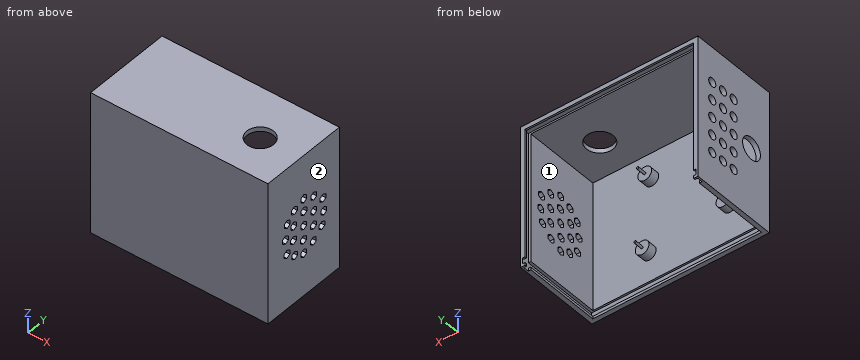
from build123d import *

# Parameters (mm, degrees)
SKETCH1_W           = 200
SKETCH1_H           = 160
BOSS_EXTRUDE1_DEPTH = 100
SHELL2_T            = -5
SKETCH2_W           = 196
SKETCH2_H           = 6.5
CUT_EXTRUDE1_DEPTH  = 97
SKETCH3_W           = 196
SKETCH3_H           = 6.2
CUT_EXTRUDE2_DEPTH  = 157
SKETCH4_R           = 15
CUT_EXTRUDE3_DEPTH  = 273.075357208
CUT_EXTRUDE4_DEPTH  = 5
SKETCH6_R           = 1.25
BOSS_EXTRUDE2_DEPTH = 20
SKETCH7_R           = 7.75
SKETCH7_R_2         = 1.25
BOSS_EXTRUDE3_DEPTH = 10
SKETCH8_R           = 12.5
SKETCH8_R_2         = 5
CUT_EXTRUDE5_DEPTH  = 5


with BuildPart() as part:
    # Sketch1 → Boss-Extrude1 (new body)
    with BuildSketch(Plane(origin=(0, 0, 0), x_dir=(1, 0, 0), z_dir=(0, 1, 0))):
        with Locations((100, 80)):
            Rectangle(SKETCH1_W, SKETCH1_H)
    extrude(amount=BOSS_EXTRUDE1_DEPTH)

    # Shell2
    shell2_openings = [part.faces().sort_by_distance(p)[0] for p in [
        (100, 100, -80),
        (100, 50, -160),
    ]]
    offset(amount=SHELL2_T, openings=shell2_openings, kind=Kind.INTERSECTION)

    # Sketch2 → Cut-Extrude1 (cut)
    with BuildSketch(Plane(origin=(0, 100, 0), x_dir=(1, 0, 0), z_dir=(0, 1, 0))):
        with Locations((100, 153.75)):
            Rectangle(SKETCH2_W, SKETCH2_H)
    extrude(amount=-CUT_EXTRUDE1_DEPTH, mode=Mode.SUBTRACT)

    # Sketch3 → Cut-Extrude2 (cut)
    with BuildSketch(Plane(origin=(0, 0, -160), x_dir=(-1, 0, 0), z_dir=(0, 0, -1))):
        with Locations((-100, 94.9)):
            Rectangle(SKETCH3_W, SKETCH3_H)
    extrude(amount=-CUT_EXTRUDE2_DEPTH, mode=Mode.SUBTRACT)

    # Sketch4 → Cut-Extrude3 (cut, through all)
    with BuildSketch(Plane(origin=(0, 0, -5), x_dir=(-1, 0, 0), z_dir=(0, 0, -1))):
        with Locations((-155, 45)):
            Circle(SKETCH4_R)
    extrude(amount=-CUT_EXTRUDE3_DEPTH, mode=Mode.SUBTRACT)

    # Sketch5 → Cut-Extrude4 (cut)
    with BuildSketch(Plane(origin=(200, 0, 0), x_dir=(0, 0, -1), z_dir=(1, 0, 0))):
        Polygon((68.441020245, 50.331851937), (66.131619168, 54.331851937), (61.512817015, 54.331851937), (59.203415938, 50.331851937), (61.512817015, 46.331851937), (66.131619168, 46.331851937), align=None)
        Polygon((84.618802154, 50), (82.309401077, 54), (77.690598923, 54), (75.381197846, 50), (77.690598923, 46), (82.309401077, 46), align=None)
        Polygon((74.50790233, 60.176296078), (76.817303407, 64.176296078), (74.50790233, 68.176296078), (69.889100176, 68.176296078), (67.5796991, 64.176296078), (69.889100176, 60.176296078), align=None)
        Polygon((86.066882085, 59.844444141), (90.685684238, 59.844444141), (92.995085315, 63.844444141), (90.685684238, 67.844444141), (86.066882085, 67.844444141), (83.757481008, 63.844444141), align=None)
        Polygon((91.558979755, 49.668148063), (93.868380832, 45.668148063), (98.487182985, 45.668148063), (100.796584062, 49.668148063), (98.487182985, 53.668148063), (93.868380832, 53.668148063), align=None)
        Polygon((85.49209767, 39.823703922), (83.182696593, 35.823703922), (85.49209767, 31.823703922), (90.110899824, 31.823703922), (92.4203009, 35.823703922), (90.110899824, 39.823703922), align=None)
        Polygon((73.933117915, 40.155555859), (69.314315762, 40.155555859), (67.004914685, 36.155555859), (69.314315762, 32.155555859), (73.933117915, 32.155555859), (76.242518992, 36.155555859), align=None)
        Polygon((57.642141445, 60.103624342), (59.951542522, 64.103624342), (57.642141445, 68.103624342), (53.023339291, 68.103624342), (50.713938215, 64.103624342), (53.023339291, 60.103624342), align=None)
        Polygon((51.720243637, 46.056331866), (54.029644713, 50.056331866), (51.720243637, 54.056331866), (47.101441483, 54.056331866), (44.792040406, 50.056331866), (47.101441483, 46.056331866), align=None)
        Polygon((56.815830123, 33.11078782), (59.1252312, 37.11078782), (56.815830123, 41.11078782), (52.197027969, 41.11078782), (49.887626893, 37.11078782), (52.197027969, 33.11078782), align=None)
        Polygon((66.04297322, 22.919614847), (68.352374296, 26.919614847), (66.04297322, 30.919614847), (61.424171066, 30.919614847), (59.114769989, 26.919614847), (61.424171066, 22.919614847), align=None)
        Polygon((82.431481108, 20.578399435), (84.740882185, 24.578399435), (82.431481108, 28.578399435), (77.812678954, 28.578399435), (75.503277878, 24.578399435), (77.812678954, 20.578399435), align=None)
        Polygon((99.921737426, 22.506459186), (102.231138502, 26.506459186), (99.921737426, 30.506459186), (95.302935272, 30.506459186), (92.993534195, 26.506459186), (95.302935272, 22.506459186), align=None)
        Polygon((108.3225692, 33.386224927), (110.631970277, 37.386224927), (108.3225692, 41.386224927), (103.703767047, 41.386224927), (101.39436597, 37.386224927), (103.703767047, 33.386224927), align=None)
        Polygon((113.969029901, 46.056331866), (116.278430978, 50.056331866), (113.969029901, 54.056331866), (109.350227748, 54.056331866), (107.040826671, 50.056331866), (109.350227748, 46.056331866), align=None)
        Polygon((108.598006308, 59.552750127), (110.907407385, 63.552750127), (108.598006308, 67.552750127), (103.979204154, 67.552750127), (101.669803077, 63.552750127), (103.979204154, 59.552750127), align=None)
        Polygon((98.574670101, 71.528102354), (100.884071178, 75.528102354), (98.574670101, 79.528102354), (93.955867948, 79.528102354), (91.646466871, 75.528102354), (93.955867948, 71.528102354), align=None)
        Polygon((83.56334775, 74.000874378), (85.872748827, 78.000874378), (83.56334775, 82.000874378), (78.944545596, 82.000874378), (76.63514452, 78.000874378), (78.944545596, 74.000874378), align=None)
        Polygon((68.276588291, 73.030682559), (70.585989368, 77.030682559), (68.276588291, 81.030682559), (63.657786138, 81.030682559), (61.348385061, 77.030682559), (63.657786138, 73.030682559), align=None)
    extrude(amount=-CUT_EXTRUDE4_DEPTH, mode=Mode.SUBTRACT)

    # Sketch6 → Boss-Extrude2 (add)
    with BuildSketch(Plane(origin=(0, 5, 0), x_dir=(1, 0, 0), z_dir=(0, 1, 0))):
        with Locations(Location((128.5, 35.2, 0), (0, 0, 90))):
            Circle(SKETCH6_R)
        with Locations(Location((131.4, 118.2, 0), (0, 0, 90))):
            Circle(SKETCH6_R)
        with Locations(Location((37.5, 31, 0), (0, 0, 90))):
            Circle(SKETCH6_R)
        with Locations(Location((40.4, 111, 0), (0, 0, 90))):
            Circle(SKETCH6_R)
    extrude(amount=BOSS_EXTRUDE2_DEPTH)

    # Sketch7 → Boss-Extrude3 (add)
    # profile 1 of 4: a face of its own
    with BuildSketch(Plane(origin=(0, 5, 0), x_dir=(1, 0, 0), z_dir=(0, 1, 0))):
        with Locations(Location((131.4, 118.2, 0), (0, 0, 90))):
            Circle(SKETCH7_R)
        with Locations(Location((131.4, 118.2, 0), (0, 0, 270))):
            Circle(SKETCH7_R_2, mode=Mode.SUBTRACT)
    # profile 2 of 4: a face of its own
    with BuildSketch(Plane(origin=(0, 5, 0), x_dir=(1, 0, 0), z_dir=(0, 1, 0))):
        with Locations(Location((40.4, 111, 0), (0, 0, 90))):
            Circle(SKETCH7_R)
        with Locations(Location((40.4, 111, 0), (0, 0, 270))):
            Circle(SKETCH7_R_2, mode=Mode.SUBTRACT)
    # profile 3 of 4: a face of its own
    with BuildSketch(Plane(origin=(0, 5, 0), x_dir=(1, 0, 0), z_dir=(0, 1, 0))):
        with Locations(Location((128.5, 35.2, 0), (0, 0, 90))):
            Circle(SKETCH7_R)
        with Locations(Location((128.5, 35.2, 0), (0, 0, 270))):
            Circle(SKETCH7_R_2, mode=Mode.SUBTRACT)
    # profile 4 of 4: a face of its own
    with BuildSketch(Plane(origin=(0, 5, 0), x_dir=(1, 0, 0), z_dir=(0, 1, 0))):
        with Locations(Location((37.5, 31, 0), (0, 0, 90))):
            Circle(SKETCH7_R)
        with Locations(Location((37.5, 31, 0), (0, 0, 270))):
            Circle(SKETCH7_R_2, mode=Mode.SUBTRACT)
    extrude(amount=BOSS_EXTRUDE3_DEPTH)

    # Sketch8 → Cut-Extrude5 (cut)
    with BuildSketch(Plane.ZY):
        with Locations((-80, 25)):
            Circle(SKETCH8_R)
        with Locations((-80, 50)):
            Circle(SKETCH8_R_2)
        with Locations((-60, 50)):
            Circle(SKETCH8_R_2)
        with Locations((-40, 50)):
            Circle(SKETCH8_R_2)
        with Locations((-60, 65)):
            Circle(SKETCH8_R_2)
        with Locations((-40, 65)):
            Circle(SKETCH8_R_2)
        with Locations((-60, 80)):
            Circle(SKETCH8_R_2)
        with Locations((-40, 80)):
            Circle(SKETCH8_R_2)
        with Locations((-80, 65)):
            Circle(SKETCH8_R_2)
        with Locations((-80, 80)):
            Circle(SKETCH8_R_2)
        with Locations((-120, 50)):
            Circle(SKETCH8_R_2)
        with Locations((-100, 50)):
            Circle(SKETCH8_R_2)
        with Locations((-120, 65)):
            Circle(SKETCH8_R_2)
        with Locations((-100, 65)):
            Circle(SKETCH8_R_2)
        with Locations((-120, 80)):
            Circle(SKETCH8_R_2)
        with Locations((-100, 80)):
            Circle(SKETCH8_R_2)
    extrude(amount=-CUT_EXTRUDE5_DEPTH, mode=Mode.SUBTRACT)


solid = part.part
The model under review builds one solid part; all positions refer to its coordinate system, in mm. Face numbers are marked on the shaded views. A direction names the side the tool comes from. Give positions to 0.01 mm unless a question says otherwise; leave off trailing zeros. Order: outer loops, then holes, each group sorted by start corner. A loop starts at its lowest first (then second) coordinate and runs counter-clockwise, first axis right, second up. Notation, with made-up numbers: M 73,56.25 L 126,56.25 A17 cw 126,60.25 Z; hole C -4,-6 d3. An arc over 180 degrees is marked long. Answer in a Markdown table with one row per item. Add a question column.
1. For pin 1 Ø1.5 at (x, z) = (79.5, -56) entering from +Y; pin 2 Ø6 at (x, y) = (72, 66.5) entering from -Z, all flat-tipped, find the tip position at first contact; note any pin that passes through.
2. Add section A-A on x = 151. State the section outline as (y, z) points, plus the area to 3 significant figures.
3. Add section B-B on x = 177. State the section outline as (y, z) points.
4. To check wall thickness, follow line 1 along Y through (x, z) = (3.95, -100); line 2 along X through (y, z) = (58.5, -36); line 3 along X through (y, z) = (92.5, -86). State the ranges of each line that lie inside material, in increasing order.
5. Machinability: for the marked faces 1 and 2, which of the approach directions +Z, -Z, +X, -X, +Y, -Y give a long, thin tool a straight path to every point of the face, cutting with its end or side? Answer none if there is none.
The answers:
| question | item | result |
|---|---|---|
| 1 | pin 1 | y = 5 |
| 1 | pin 2 | z = -5 |
| 2 | outline | M 0,-160 L 5,-160 L 5,-157 L 3,-157 L 3,-150.5 L 5,-150.5 L 5,-5 L 30.54,-5 L 30.54,0 L 0,0 Z; M 59.46,-5 L 91.8,-5 L 91.8,-3 L 98,-3 L 98,-5 L 100,-5 L 100,0 L 59.46,0 Z |
| 2 | area | 1,110 mm2 |
| 3 | outline | M 0,-160 L 5,-160 L 5,-157 L 3,-157 L 3,-150.5 L 5,-150.5 L 5,-5 L 91.8,-5 L 91.8,-3 L 98,-3 L 98,-5 L 100,-5 L 100,0 L 0,0 Z |
| 4 | line 1 | 0 to 45, 55 to 60, 70 to 75, 85 to 91.8, 98 to 100 |
| 4 | line 2 | 0 to 5, 195 to 200 |
| 4 | line 3 | 0 to 2, 198 to 200 |
| 5 | face 1 | -Z, +Y |
| 5 | face 2 | +Z, -Z, +X, +Y, -Y |
